For this review, take the finished solid that the model builds, in its own axes (mm). A direction names the side the tool comes from. Give positions to 0.01 mm unless a question says otherwise; leave off trailing zeros. Order: outer loops, then holes, each group sorted by start corner. A loop starts at its lowest first (then second) coordinate and runs counter-clockwise, first axis right, second up.
Item 1: Consider section C-C (x = 5.5). Give the boundary of the cut face in (y, z), plus the area to 3 significant figures.
Item 2: For P1, Ø1.5, axis at y = -1.5, z = 1.5, coming from the -X side; P2, Ø3, axis at x = -2, y = 0, coming from the -Z side; P3, Ø1, axis at x = -4.5, z = 2.5, coming from the -Y side; P4, Ø2, axis at y = 8, z = 0.5, coming from the +X side, all flat-tipped, find the tip position at first contact; note any pin that passes through.
Item 3: Consider section A-A (x = 0). Give the boundary of the cut face in (y, z), plus the area to 3 significant figures.
Item 4: Machinability: for faces 4 (the flat face through (-3.46, 9.33, 2.58)), 5 (the flat face through (9.901, 0.734, 2.576)), 6 (the flat face through (-4.78, 8.7, 2.58)), which of the approach directions +Z, -Z, +X, -X, +Y, -Y give a long, thin tool a straight path to every point of the face, cutting with its end or side? Answer none if there is none.
Item 5: Consider section B-B (y = 3). Give the boundary of the cut face in (x, z) (3 decimals).
Item 6: For probe 1 along Y at (x, z) = (6.75, 3.6); probe 2 along X at (y, z) = (-1.25, 4.2) (3 decimals); probe 3 along Y at (x, z) = (8.5, 1.25), list the stretches that pass through material, from the lowest coordinate up.
Item 7: The part is to be moulded in two halves that separate along X. For faces 1 (the flat face through (-9.707, 2.085, 2.576)), 2 (the flat face through (-5.95, 7.98, 2.58)), 3 (the flat face through (9.73, 2.1, 2.58)), say which applies: released by +X, released by -X, zero draft, split by the parting line, or undercut.
```python
from build123d import *

# Parameters (mm, degrees)
F0_R            = 10.909800859
F1_DEPTH        = 5.08
F3_DEPTH        = 5.08
F3_COPIES_COUNT = 22


# Not quite as in the source:
# - a pattern or mirror of a feature is missing from the dataset's text; its kind, count and spacing are read off the source's solid


with BuildPart() as f1:
    # F0 (on Top) → F1 (new body)
    with BuildSketch(Plane.XY):
        Circle(F0_R)
        with BuildLine():
            ThreePointArc((3.8749986, -3.9031251389), (0, -5.5), (-3.8749986, -3.9031251389))
            Line((-3.8749986, -3.9031251389), (-3.8749986, 3.9031251389))
            ThreePointArc((-3.8749986, 3.9031251389), (0, 5.5), (3.8749986, 3.9031251389))
            Line((3.8749986, 3.9031251389), (3.8749986, -3.9031251389))
        make_face(mode=Mode.SUBTRACT)
    extrude(amount=F1_DEPTH)

    # F2 (on face) → F3 (cut, through all)
    with BuildSketch(Plane.XY.offset(5.08)):
        with BuildLine():
            Line((0.2718847261, 8.9821943232), (1.1039126824, 10.8538072386))
            ThreePointArc((1.1039126824, 10.8538072386), (0, 10.909800859), (-1.1039126824, 10.8538072386))
            Line((-1.1039126824, 10.8538072386), (-0.2718847261, 8.9821943232))
            ThreePointArc((-0.2718847261, 8.9821943232), (0, 8.8055210085), (0.2718847261, 8.9821943232))
        make_face()
    f3 = extrude(amount=-F3_DEPTH, mode=Mode.SUBTRACT)

    # F3_copies: F3 ×22 about axis
    f3_copies_axis = Axis((0, 0, 0), (0, 0, 1))
    for i in range(1, F3_COPIES_COUNT):
        add(f3.rotate(f3_copies_axis, i * 360 / F3_COPIES_COUNT), mode=Mode.SUBTRACT)


solid = f1.part
```
Resolved:
1. outline: (-7.68, 0) - (7.68, 0) - (7.68, 5.08) - (-7.68, 5.08) - close
1. area: 78.0 mm2
2. P1: stops at x = -9.97
2. P2: passes through
2. P3: stops at y = -10.1
2. P4: stops at x = 7.48
3. outline: (-8.81, 0) - (-5.5, 0) - (-5.5, 5.08) - (-8.81, 5.08) - close; (5.5, 0) - (8.81, 0) - (8.81, 5.08) - (5.5, 5.08) - close
3. area: 33.6 mm2
4. face 4: +Z, -Z, +Y
4. face 5: +Z, -Z, +X
4. face 6: +Z, -Z
5. outline: (-10.489, 0) - (-3.875, 0) - (-3.875, 5.08) - (-10.489, 5.08) - close; (3.875, 0) - (10.489, 0) - (10.489, 5.08) - (3.875, 5.08) - close
6. probe 1: y = -8.5 to -6.39, -5.69 to 5.69, 6.39 to 8.5
6. probe 2: x = -8.716 to -3.875, 3.875 to 8.716
6. probe 3: y = -6.14 to -4.48, -3.49 to 3.49, 4.48 to 6.14
7. face 1: released by -X
7. face 2: undercut
7. face 3: released by +X
